Check sheet for the modelled part. Datum: model origin and axes. Units: mm. A direction names the side the tool comes from. Round coordinates to 2 decimals unless told otherwise and drop trailing zeros. Write each loop counter-clockwise with the first axis right and the second up, starting at its lowest first coordinate (ties: lowest second). Pieces come first, ordered by that corner, then holes.
Item 1: Cross-section at C-C on z = 3.75. Enter the section's corners in (x, y), plus the area to 3 significant figures.
Item 2: Go/stop test with a flat-tipped pin: pin 1 Ø1.5 at (y, z) = (3, 3.5) entering from +X. Record where the tip stops, or that it passes through.
Item 3: Cross-section at B-B on y = 3. Enter the section's corners in (x, z), plus the area to 3 significant figures.
Item 4: Cross-section at D-D on y = 0.95. Enter the section's corners in (x, z), plus the area to 3 significant figures.
Item 5: Material ranges on line 1 (Z direction, x = -3.3, y = 0.5); line 2 (X direction, y = 3.6, z = 3.6); line 3 (X direction, y = 4.15, z = 3.1), recorded low to high.
Item 6: Tool access check on faces 1 (the flat face through (-3, 3, 4)), 2 (the flat face through (-4.4, 4.4, 3)). Record the directions out of +Z, -Z, +X, -X, +Y, -Y that give a thin tool (end or side, any length) a straight path to the whole face; none if there is none.
Item 7: Cross-section at A-A on x = -3. Enter the section's corners in (y, z), plus the area to 3 significant figures.
from build123d import *

# Parameters (mm, degrees)
SKETCH_1_W      = 6
SKETCH_1_H      = 6
SKETCH_1_R      = 1.5
EXTRUDE_1_DEPTH = 3
SKETCH_1_3_R    = 1.5
EXTRUDE_2_DEPTH = 4


with BuildPart() as part:
    # Sketch 1 → Extrude 1 (new body)
    # profile 1 of 2: a face of its own
    with BuildSketch(Plane.XY):
        with Locations((-3, 3)):
            Rectangle(SKETCH_1_W, SKETCH_1_H)
        with Locations((-3, 3)):
            Circle(SKETCH_1_R, mode=Mode.SUBTRACT)
    # profile 2 of 2: a face of its own
    with BuildSketch(Plane.XY):
        with Locations((-3, 3)):
            Circle(SKETCH_1_R)
    extrude(amount=EXTRUDE_1_DEPTH)

    # Sketch 1_3 → Extrude 2 (add)
    with BuildSketch(Plane.XY):
        with Locations((-3, 3)):
            Circle(SKETCH_1_3_R)
    extrude(amount=EXTRUDE_2_DEPTH)


solid = part.part
Response values:
1. outline: circle Ø3 at (-3, 3)
1. area: 7.07 mm2
2. pin 1: stops at x = 0
3. outline: (-6, 0) - (0, 0) - (0, 3) - (-1.5, 3) - (-1.5, 4) - (-4.5, 4) - (-4.5, 3) - (-6, 3) - close
3. area: 21.0 mm2
4. outline: (-6, 0) - (0, 0) - (0, 3) - (-6, 3) - close
4. area: 18.0 mm2
5. line 1: z = 0 to 3
5. line 2: x = -4.37 to -1.63
5. line 3: x = -3.96 to -2.04
6. face 1: +Z, +X, -X, +Y, -Y
6. face 2: +Z
7. outline: (0, 0) - (6, 0) - (6, 3) - (4.5, 3) - (4.5, 4) - (1.5, 4) - (1.5, 3) - (0, 3) - close
7. area: 21.0 mm2
